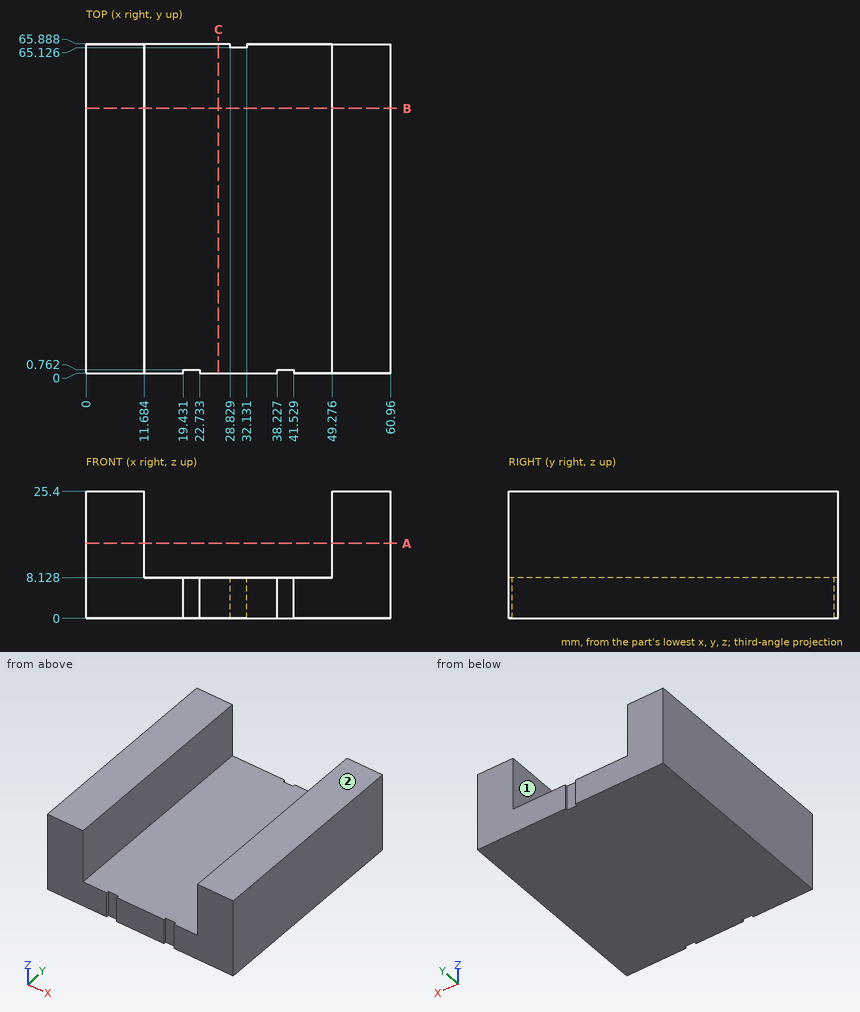
Part print with two shaded views. Sizes in mm from the minimum x, y, z corner. A direction names the side the tool comes from. Round coordinates to 2 decimals unless told otherwise and drop trailing zeros. Loops run counter-clockwise (first coordinate to the right, second up) from the corner with the lowest first, then second, coordinate; pieces in that order, holes last.
1. Flat gauge pins, fed straight in: pin 1 (6 mm diameter, centred on x = 19.5, y = 16, fed in from +Z); pin 2 (1 mm diameter, centred on x = 40, z = 4.5, fed in from -Y). Where does each tip first touch, or does it go through?
Solutions:
pin 1: stops at z = 8.13
pin 2: stops at y = 0.76
2. Slice it at A-A (z = 15). Give the cut face in (x, y).
Solutions:
outline: (0, 0) - (11.68, 0) - (11.68, 65.89) - (0, 65.89) - close; (49.28, 0) - (60.96, 0) - (60.96, 65.89) - (49.28, 65.89) - close
3. Slice it at B-B (y = 53). Give the cut face in (x, z).
Solutions:
outline: (0, 0) - (60.96, 0) - (60.96, 25.4) - (49.28, 25.4) - (49.28, 8.13) - (11.68, 8.13) - (11.68, 25.4) - (0, 25.4) - close
4. 3-axis set-ups, long thin cutter, end or side, ignore diameter. For the marked faces 1 and 2: which of +Z, -Z, +X, -X, +Y, -Y reach the whole face in a straight line?
Solutions:
face 1: +Z, +Y, -Y
face 2: +Z, +X, -X, +Y, -Y
5. Slice it at C-C (x = 26.5). Give the cut face in (y, z).
Solutions:
outline: (0, 0) - (65.89, 0) - (65.89, 8.13) - (0, 8.13) - close
6. Drill centre lines: line 1 along X through (y, z) = (29.5, 21.5); line 2 along Z through (x, y) = (43, 36). Where is each one in solid material? Low to high.
Solutions:
line 1: x = 0 to 11.68, 49.28 to 60.96
line 2: z = 0 to 8.13
